from build123d import *

# Parameters (mm, degrees)
F0_R     = 5
F1_DEPTH = 1.25
F2_DEPTH = 12.5
F3_DEPTH = 12.5


with BuildPart() as f1:
    # F0 (on Front) → F1 (new body, symmetric)
    with BuildSketch(Plane.XZ):
        with BuildLine():
            ThreePointArc((0, 20), (-10, 10), (0, 0))
            Line((0, 0), (30, 0))
            ThreePointArc((30, 0), (40, 10), (30, 20))
            Line((30, 20), (0, 20))
        make_face()
        with Locations((0, 10)):
            Circle(F0_R, mode=Mode.SUBTRACT)
        with Locations((30, 10)):
            Circle(F0_R, mode=Mode.SUBTRACT)
        with Locations((30, 10)):
            Circle(F0_R)
        with Locations((0, 10)):
            Circle(F0_R)
    extrude(amount=F1_DEPTH, both=True)

    # F0 (on Front) → F2 (join)
    with BuildSketch(Plane.XZ):
        with Locations((0, 10)):
            Circle(F0_R)
    extrude(amount=F2_DEPTH)

    # F0 (on Front) → F3 (join)
    with BuildSketch(Plane.XZ):
        with Locations((30, 10)):
            Circle(F0_R)
    extrude(amount=-F3_DEPTH)


solid = f1.part
Build history of the part. All positions in model axes, mm. A direction names the side the tool comes from. Round coordinates to 2 decimals unless told otherwise and drop trailing zeros. Write each loop counter-clockwise with the first axis right and the second up, starting at its lowest first coordinate (ties: lowest second). Pieces come first, ordered by that corner, then holes. Notation, with made-up numbers: M 48,-17 L 93,-17 A13 ccw 93,-4 Z; hole C 19.5,62.25 d5. An arc over 180 degrees is marked long. Answer as a JSON object with one key per item and string values. Group by question number.
(1) Flat gauge pins, fed straight in: pin 1 (6 mm diameter, centred on x = 3.5, z = 6, fed in from +Y); pin 2 (12 mm diameter, centred on y = -9.5, z = 8, fed in from +X); pin 3 (8 mm diameter, centred on y = 3.5, z = 17.5, fed in from -X). Where does each tip first touch, or does it go through?
(2) Drill centre lines: L1, parallel to Y at x = 21.5, z = 8.5; L2, parallel to Y at x = -1, z = 14; L3, parallel to X at y = 8.25, z = 8.25. Where is each one in solid material? Low to high.
(3) Cut at D-D (z = 4). Give the cut face in (x, y), and give its area (3 significant figures).
(4) Cut at A-A (z = 10). Give the cut face in (x, y).
(5) Which spindle directions (+Z, -Z, +X, -X, +Y, -Y) get a long thin tool onto all of the face, cutting with end or side? Do faces 1 (the cylindrical face through (-0.651, -6.796, 14.957)), 2 (the cylindrical face through (40, 0, 10)), 3 (the cylindrical face through (25, 7, 10)). Say none if no direction does.
(6) Cut at B-B (y = 5.5). Give the cut face in (x, z).
(7) Cut at C-C (x = 17.5). Give the cut face in (y, z).
Responses:
{
 "1": {"pin 1": "stops at y = 1.25", "pin 2": "stops at x = 5", "pin 3": "stops at x = -9.08"},
 "2": {"L1": "y = -1.25 to 1.25", "L2": "y = -12.5 to 1.25", "L3": "x = 25.32 to 34.68"},
 "3": {"outline": "M -8,-1.25 L 38,-1.25 L 38,1.25 L -8,1.25 Z", "area": "115 mm2"},
 "4": {"outline": "M -10,-1.25 L -5,-1.25 L -5,-12.5 L 5,-12.5 L 5,-1.25 L 40,-1.25 L 40,1.25 L 35,1.25 L 35,12.5 L 25,12.5 L 25,1.25 L -10,1.25 Z"},
 "5": {"face 1": "-Y", "face 2": "+X, +Y, -Y", "face 3": "+Y"},
 "6": {"outline": "C 30,10 d10"},
 "7": {"outline": "M -1.25,0 L 1.25,0 L 1.25,20 L -1.25,20 Z"}
}
